Solid Edge part; units mm, degrees
sketch "Sketch1" plane through (0, 0, 0) normal (0, -1, 0) x (1, 0, 0)
  line L0 (60, -30) -> (60, 30)
  line L1 (60, 30) -> (-60, 30)
  line L2 (-60, 30) -> (-60, -30)
  line L3 (-60, -30) -> (60, -30)
extrude "Protrusion1" add sketch "Sketch1" against normal blind 47
sketch "Sketch2" plane through (60, 23.5, 0) normal (1, 0, 0) x (0, 1, 0)
  line L0 (-23.5, 30) -> (-23.5, 27.5)
  line L1 (-23.5, 27.5) -> (20.5, 27.5)
  line L2 (20.5, 27.5) -> (20.5, 30)
  line L3 (20.5, 30) -> (-23.5, 30)
extrude "ExtrudedCutout_1" cut sketch "Sketch2" against normal blind 121
sketch "Sketch3" plane through (60, 23.5, 0) normal (1, 0, 0) x (0, 1, 0)
  line L0 (-23.5, -30) -> (-23.5, -27.5)
  line L1 (-23.5, -27.5) -> (20.5, -27.5)
  line L2 (20.5, -27.5) -> (20.5, -30)
  line L3 (20.5, -30) -> (-23.5, -30)
extrude "ExtrudedCutout_2" cut sketch "Sketch3" against normal blind 121
sketch "Sketch4" plane through (60, 23.5, 0) normal (1, 0, 0) x (0, 1, 0)
  circle A0 centre (1.45, 27.5) radius 19.05
extrude "ExtrudedCutout_3" cut sketch "Sketch4" against normal blind 121
sketch "Sketch5" plane through (60, 23.5, 0) normal (1, 0, 0) x (0, 1, 0)
  circle A0 centre (1.45, -27.5) radius 19.05
extrude "ExtrudedCutout_5" cut sketch "Sketch5" against normal blind 121
sketch "Sketch6" plane through (60, 23.5, 0) normal (1, 0, 0) x (0, 0, -1)
  line L0 (-27.5, -23.5) -> (-15, -23.5)
  line L1 (-15, -23.5) -> (-15, -18.5)
  line L2 (-15, -18.5) -> (15, -18.5)
  line L3 (15, -18.5) -> (15, -23.5)
  line L4 (15, -23.5) -> (27.5, -23.5)
extrude "ExtrudedCutout_6" cut sketch "Sketch6" against normal blind 120 material side at (60, -0.05, 21.25)
sketch "Sketch7" plane through (0, 5, 0) normal (0, -1, 0) x (1, 0, 0)
  circle A0 centre (0, 0) radius 6
extrude "ExtrudedCutout_7" cut sketch "Sketch7" against normal blind 47
sketch "Sketch8" plane through (0, 5, 0) normal (0, -1, 0) x (1, 0, 0)
  circle A0 centre (0, 0) radius 8
extrude "ExtrudedCutout_8" cut sketch "Sketch8" against normal blind 5
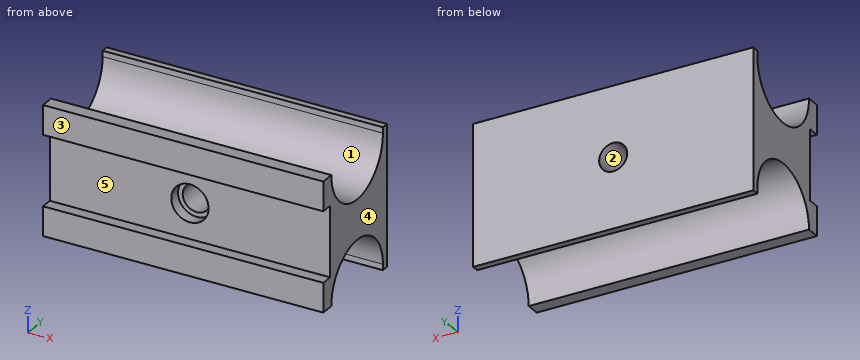
Check sheet for the modelled part. Datum: model origin and axes. Units: mm. Face numbers are marked on the shaded views. A direction names the side the tool comes from. Coordinates: 2 decimals unless noted, no trailing zeros. Write each loop counter-clockwise with the first axis right and the second up, starting at its lowest first coordinate (ties: lowest second). Pieces come first, ordered by that corner, then holes. Notation, with made-up numbers: (29, 35.25) -> (53, 35.25) arc R27 cw to (53, 60.25) -> close; hole circle Ø8 at (44, -39.5). An arc over 180 degrees is marked (long way). Use a Markdown table: item, result.
1. Go/stop test with flat-tipped pins: pin 1 Ø14.5 at (x, z) = (0, 0) entering from -Y; pin 2 Ø1.5 at (x, y) = (-12, 33.5) entering from -Z; pin 3 Ø9 at (x, z) = (19, 2) entering from -Y. Record where each tip stops, or that it passes through.
Reported:
| item | result |
|---|---|
| pin 1 | stops at y = 10 |
| pin 2 | stops at z = -10.87 |
| pin 3 | stops at y = 5 |
2. Sectioned sample at D-D (y = 29.5). Enter the section's corners in (x, z), plus the area to 3 significant figures.
Reported:
| item | result |
|---|---|
| outline | (-60, -9) -> (60, -9) -> (60, 9) -> (-60, 9) -> close; hole circle Ø12 at (0, 0) |
| area | 2,050 mm2 |
3. Release check for a two-part mould opening along Z. For the marked faces 1, 2 and 3 record: pulls with the +Z half, pulls with the -Z half, needs draft (parallel to the pull), parting line crosses it, or undercut.
Reported:
| item | result |
|---|---|
| face 1 | pulls with the +Z half |
| face 2 | undercut |
| face 3 | needs draft |
4. Sectioned sample at C-C (x = -26). Enter the section's corners in (y, z), plus the area to 3 significant figures.
Reported:
| item | result |
|---|---|
| outline | (0, -27.5) -> (5.9, -27.5) arc R19.05 cw to (44, -27.5) -> (44, -30) -> (47, -30) -> (47, 30) -> (44, 30) -> (44, 27.5) arc R19.05 cw to (5.9, 27.5) -> (0, 27.5) -> (0, 15) -> (5, 15) -> (5, -15) -> (0, -15) -> close |
| area | 1,310 mm2 |
5. Sectioned sample at A-A (z = 0). Enter the section's corners in (x, y).
Reported:
| item | result |
|---|---|
| outline | (-60, 5) -> (-8, 5) -> (-8, 10) -> (-6, 10) -> (-6, 47) -> (-60, 47) -> close; (6, 10) -> (8, 10) -> (8, 5) -> (60, 5) -> (60, 47) -> (6, 47) -> close |
6. Sectioned sample at B-B (x = 0). Enter the section's corners in (y, z), plus the area to 3 significant figures.
Reported:
| item | result |
|---|---|
| outline | (0, -27.5) -> (5.9, -27.5) arc R19.05 cw to (44, -27.5) -> (44, -30) -> (47, -30) -> (47, -6) -> (10, -6) -> (10, -8) -> (5, -8) -> (5, -15) -> (0, -15) -> close; (0, 15) -> (5, 15) -> (5, 8) -> (10, 8) -> (10, 6) -> (47, 6) -> (47, 30) -> (44, 30) -> (44, 27.5) arc R19.05 cw to (5.9, 27.5) -> (0, 27.5) -> close |
| area | 786 mm2 |
7. Tool access check on the marked faces 4 and 5. Record the directions out of +Z, -Z, +X, -X, +Y, -Y that give a thin tool (end or side, any length) a straight path to the whole face; none if there is none.
Reported:
| item | result |
|---|---|
| face 4 | +Z, -Z, +X, +Y, -Y |
| face 5 | +X, -X, -Y |
8. Scan lines: line 1 along Z through (x, y) = (0, 25); line 2 along Z through (x, y) = (-32, 4); line 3 along Y through (x, z) = (41, 6.5). Record each from-to range of solid material in increasing order.
Reported:
| item | result |
|---|---|
| line 1 | z = -8.45 to -6, 6 to 8.45 |
| line 2 | z = -27.5 to -15, 15 to 27.5 |
| line 3 | y = 5 to 47 |
